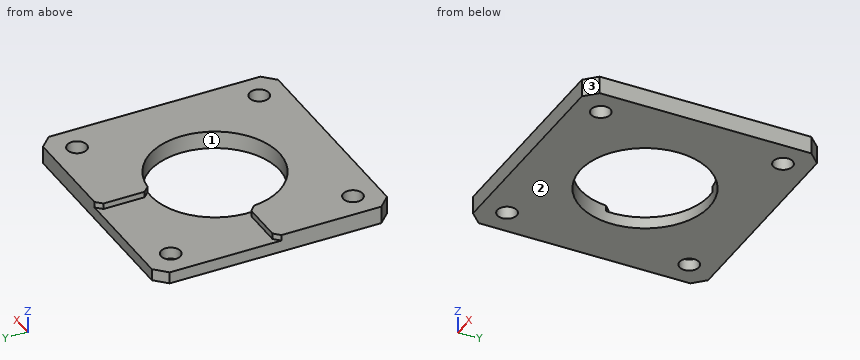
from build123d import *

# Parameters (mm, degrees)
SKETCH_W        = 40
SKETCH_H        = 40
PAD_DEPTH       = 3
SKETCH001_R     = 10.99
SKETCH001_R_2   = 1.65
POCKET_DEPTH    = 5
SKETCH003_W     = 37.54295
SKETCH003_H     = 30.927837
POCKET001_DEPTH = 1
CHAMFER_SIZE    = 2
CHAMFER001_SIZE = 1


with BuildPart() as part:
    # Sketch → Pad (new body)
    with BuildSketch(Plane.XY):
        Rectangle(SKETCH_W, SKETCH_H)
    extrude(amount=PAD_DEPTH)

    # Sketch001 (on Face6 of Pad) → Pocket (cut)
    with BuildSketch(Plane.XY.offset(3)):
        Circle(SKETCH001_R)
        with Locations((-15.5, 15.5)):
            Circle(SKETCH001_R_2)
        with Locations((15.5, 15.5)):
            Circle(SKETCH001_R_2)
        with Locations((-15.5, -15.5)):
            Circle(SKETCH001_R_2)
        with Locations((15.5, -15.5)):
            Circle(SKETCH001_R_2)
    extrude(amount=-POCKET_DEPTH, mode=Mode.SUBTRACT)

    # Sketch003 (on Face5 of Pocket) → Pocket001 (cut)
    with BuildSketch(Plane.XY.offset(3)):
        with Locations((-18.771475, 15.463919)):
            Rectangle(SKETCH003_W, SKETCH003_H)
    extrude(amount=-POCKET001_DEPTH, mode=Mode.SUBTRACT)

    # Chamfer
    chamfer_edges = [part.edges().sort_by_distance(p)[0] for p in [
        (-20, -20, 1.5),
        (20, -20, 1.5),
        (20, 20, 1.5),
        (-20, 20, 1),
    ]]
    chamfer(chamfer_edges, length=CHAMFER_SIZE)

    # Chamfer001
    chamfer001_edges = [part.edges().sort_by_distance(p)[0] for p in [
        (-10.99, 0, 2.5),
        (0, 20, 2.5),
        (0, 10.99, 2.5),
        (-20, 0, 2.5),
    ]]
    chamfer(chamfer001_edges, length=CHAMFER001_SIZE)


solid = part.part
Work out the finished part from the listing and answer in its coordinate system (mm). Face numbers are marked on the shaded views. Round coordinates to 2 decimals unless told otherwise and drop trailing zeros. Write each loop counter-clockwise with the first axis right and the second up, starting at its lowest first coordinate (ties: lowest second). Pieces come first, ordered by that corner, then holes. Notation, with made-up numbers: (12.5, 2.5) - (22.5, 2.5) arc R9 cw to (22.5, 8.5) - close; hole circle Ø6 at (46.5, -23). An arc over 180 degrees is marked (long way). Answer in a Markdown table with one row per item. Add a question column.
1. Find the intervals of material crossed by line 1 along Y through (x, z) = (15.5, 1.1); line 2 along Y through (x, z) = (0, 1.95); line 3 along X through (y, z) = (-14.5, 0.9), in increasing order. Write a range as from..to.
2. A cutting plane is placed at D-D, the plane x = -10. Determine the outline of the cut face in (y, z), and give its area (3 significant figures).
3. A cutting plane is placed at A-A, the plane x = 15.5. Determine the outline of the cut face in (y, z), and give its area (3 significant figures).
4. Given pin 1 (6.5 mm diameter, centred on x = -14, y = 10.5, fed in from +Z); pin 2 (0.5 mm diameter, centred on y = 16, z = 2.5, fed in from -X); pin 3 (4 mm diameter, centred on x = -11, y = 0, fed in from +Z), each flat-ended and moving along its own axis, determine where each tip first touches the part or whether it passes through.
5. A cutting plane is placed at C-C, the plane z = 1.4. Determine the outline of the cut face in (x, y), and give its area (3 significant figures).
6. The mould has two halves that part along X. Classify the marked faces 1, 2 and 3: +X half, -X half, draft (parallel to the pull), parting line (faces both ways), or undercut.
Worked out:
| question | item | result |
|---|---|---|
| 1 | line 1 | -20..-17.15, -13.85..13.85, 17.15..20 |
| 1 | line 2 | -20..-10.99, 10.99..20 |
| 1 | line 3 | -20..-16.81, -14.19..14.19, 16.81..20 |
| 2 | outline | (-20, 0) - (-4.56, 0) - (-4.56, 3) - (-20, 3) - close; (4.56, 0) - (20, 0) - (20, 2) - (4.56, 2) - close |
| 2 | area | 77.2 mm^2 |
| 3 | outline | (-20, 0) - (-17.15, 0) - (-17.15, 3) - (-20, 3) - close; (-13.85, 0) - (13.85, 0) - (13.85, 3) - (-13.85, 3) - close; (17.15, 0) - (20, 0) - (20, 3) - (17.15, 3) - close |
| 3 | area | 100 mm^2 |
| 4 | pin 1 | z = 2 |
| 4 | pin 2 | x = 0 |
| 4 | pin 3 | z = 3 |
| 5 | outline | (-20, -18) - (-18, -20) - (18, -20) - (20, -18) - (20, 18) - (18, 20) - (-18, 20) - (-20, 18) - close; hole circle Ø3.3 at (-15.5, -15.5); hole circle Ø3.3 at (-15.5, 15.5); hole circle Ø21.98 at (0, 0); hole circle Ø3.3 at (15.5, -15.5); hole circle Ø3.3 at (15.5, 15.5) |
| 5 | area | 1,180 mm^2 |
| 6 | face 1 | undercut |
| 6 | face 2 | draft |
| 6 | face 3 | +X half |
